Check sheet for the modelled part. Datum: model origin and axes. Units: mm. A direction names the side the tool comes from. Round coordinates to 2 decimals unless told otherwise and drop trailing zeros. Write each loop counter-clockwise with the first axis right and the second up, starting at its lowest first coordinate (ties: lowest second). Pieces come first, ordered by that corner, then holes.
Item 1: Set-up check for faces 1 (the flat face through (12, 13, -21.377)), 2 (the flat face through (12, 13, 23.219)), 3 (the cylindrical face through (-16.913, 12.522, 0.431)): record each of +Z, -Z, +X, -X, +Y, -Y from which the full face is reachable in a straight line by a thin tool's end or side.
Item 2: Depth check by flat-ended pin: pin 1 (10 mm diameter, centred on x = 9, y = 15, fed in from -Z); pin 2 (4 mm diameter, centred on x = 10.5, y = 8.5, fed in from +Z); pin 3 (2 mm diameter, centred on x = -6.5, z = 14, fed in from -Y); pin 4 (8 mm diameter, centred on x = -6.5, y = 4, fed in from -Z). Enter the tip coordinate at first touch or a pass-through.
Item 3: Section check B-B, the plane y = 11.5. Record the cut outline in (x, z).
Item 4: Section check A-A, the plane x = 10. Record the cut outline in (y, z), plus the area to 3 significant figures.
Item 5: Section check D-D, the plane x = -10. Record the cut outline in (y, z), plus the area to 3 significant figures.
Item 6: Section check C-C, the plane z = 3. Record the cut outline in (x, y), plus the area to 3 significant figures.
Item 7: Material ranges on line 1 along Z through (x, y) = (15, 5); line 2 along Y through (x, z) = (16, 23.5); line 3 along X through (y, z) = (10.5, -18), recorded low to high.
from build123d import *

# Parameters (mm, degrees)
BOSS_EXTRUDE1_DEPTH = 28
BOSS_EXTRUDE2_START = -2.6
BOSS_EXTRUDE2_DEPTH = 2.6


with BuildPart() as part:
    # Sketch1 → Boss-Extrude1 (new body)
    with BuildSketch(Plane(origin=(0, 0, 0), x_dir=(1, 0, 0), z_dir=(0, 1, 0))):
        with BuildLine():
            Line((5.379822255, -23.218858624), (17.981010255, -23.218858624))
            Line((17.981010255, -23.218858624), (17.981010255, 21.376607386))
            Line((17.981010255, 21.376607386), (5.379822255, 21.376607386))
            ThreePointArc((5.379822255, 21.376607386), (-16.91791075, -0.921125619), (5.379822255, -23.218858624))
        make_face()
    extrude(amount=BOSS_EXTRUDE1_DEPTH)

    # Sketch2 → Boss-Extrude2 (add)
    with BuildSketch(Plane(origin=(0, 28, 0), x_dir=(1, 0, 0), z_dir=(0, 1, 0)).offset(BOSS_EXTRUDE2_START)):
        with BuildLine():
            Line((5.379822255, -25.218858624), (17.981010255, -25.218858624))
            Line((17.981010255, -25.218858624), (17.981010255, -23.218858624))
            Line((17.981010255, -23.218858624), (5.379822255, -23.218858624))
            ThreePointArc((5.379822255, -23.218858624), (-16.91791075, -0.921125619), (5.379822255, 21.376607386))
            Line((5.379822255, 21.376607386), (17.981010255, 21.376607386))
            Line((17.981010255, 21.376607386), (17.981010255, 23.376607386))
            Line((17.981010255, 23.376607386), (5.379822255, 23.376607386))
            ThreePointArc((5.379822255, 23.376607386), (-18.91791075, -0.921125619), (5.379822255, -25.218858624))
        make_face()
    extrude(amount=BOSS_EXTRUDE2_DEPTH)


solid = part.part
Values found:
1. face 1: -Z, +X, -X, -Y
1. face 2: +Z, +X, -X, -Y
1. face 3: -X, -Y
2. pin 1: stops at z = -21.38
2. pin 2: stops at z = 23.22
2. pin 3: stops at y = 0
2. pin 4: stops at z = -19.94
3. outline: (5.38, -21.38) - (17.98, -21.38) - (17.98, 23.22) - (5.38, 23.22) arc R22.3 ccw to start
4. outline: (0, -21.38) - (25.4, -21.38) - (25.4, -23.38) - (28, -23.38) - (28, 25.22) - (25.4, 25.22) - (25.4, 23.22) - (0, 23.22) - close
4. area: 1,260 mm2
5. outline: (0, -15.22) - (25.4, -15.22) - (25.4, -17.89) - (28, -17.89) - (28, 19.73) - (25.4, 19.73) - (25.4, 17.07) - (0, 17.07) - close
5. area: 918 mm2
6. outline: (-18.83, 25.4) - (-16.82, 25.4) - (-16.82, 0) - (17.98, 0) - (17.98, 28) - (-18.83, 28) - close
6. area: 980 mm2
7. line 1: z = -21.38 to 23.22
7. line 2: y = 25.4 to 28
7. line 3: x = -6.42 to 17.98
